```python
from build123d import *

# Parameters (mm, degrees)
SKETCH1_W           = 50
SKETCH1_H           = 40
BOSS_EXTRUDE1_DEPTH = 10
SKETCH5_W           = 6
SKETCH5_H           = 5
BOSS_EXTRUDE3_DEPTH = 10
SKETCH6_R           = 2
CUT_EXTRUDE1_DEPTH  = 20
SKETCH8_W           = 10
SKETCH8_H           = 40
CUT_EXTRUDE2_DEPTH  = 25
SKETCH12_W          = 5
SKETCH12_H          = 5
BOSS_EXTRUDE5_DEPTH = 10
SKETCH13_R          = 1.5
CUT_EXTRUDE4_DEPTH  = 10
SKETCH14_R          = 1
CUT_EXTRUDE5_DEPTH  = 10
CUT_EXTRUDE6_DEPTH  = 22
CUT_EXTRUDE7_DEPTH  = 30
CUT_EXTRUDE8_DEPTH  = 30


with BuildPart() as part:
    # Sketch1 → Boss-Extrude1 (new body)
    with BuildSketch(Plane(origin=(669.84184187, 0, 0), x_dir=(1, 0, 0), z_dir=(0, 0, 1))):
        with Locations((-671.310344828, 437.637931034)):
            Rectangle(SKETCH1_W, SKETCH1_H)
    boss_extrude1 = extrude(amount=BOSS_EXTRUDE1_DEPTH)

    # Sketch5 → Boss-Extrude3 (add)
    with BuildSketch(Plane(origin=(23.531497042, 0, 0), x_dir=(0, 0, -1), z_dir=(1, 0, 0))):
        with Locations((-5, 442.637931034)):
            Rectangle(SKETCH5_W, SKETCH5_H)
        with Locations((-5, 432.637931034)):
            Rectangle(SKETCH5_W, SKETCH5_H)
    boss_extrude3 = extrude(amount=BOSS_EXTRUDE3_DEPTH)

    # Sketch6 → Cut-Extrude1 (cut)
    with BuildSketch(Plane(origin=(669.84184187, 445.137931034, 0), x_dir=(1, 0, 0), z_dir=(0, 1, 0))):
        with Locations(Location((-641.310344828, -5, 0), (0, 0, 180))):
            Circle(SKETCH6_R)
    cut_extrude1 = extrude(amount=-CUT_EXTRUDE1_DEPTH, mode=Mode.SUBTRACT)

    # Sketch8 → Cut-Extrude2 (cut)
    with BuildSketch(Plane.ZY.offset(26.468502958)):
        with Locations((5, 437.637931034)):
            Rectangle(SKETCH8_W, SKETCH8_H)
    extrude(amount=-CUT_EXTRUDE2_DEPTH, mode=Mode.SUBTRACT)

    # Mirror1: Boss-Extrude1, Boss-Extrude3, Cut-Extrude1 across plane
    add(boss_extrude1.mirror(Plane(origin=(-1.468502958, 0, 0), x_dir=(0, 0, 1), z_dir=(1, 0, 0))))
    add(boss_extrude3.mirror(Plane(origin=(-1.468502958, 0, 0), x_dir=(0, 0, 1), z_dir=(1, 0, 0))))
    add(cut_extrude1.mirror(Plane(origin=(-1.468502958, 0, 0), x_dir=(0, 0, 1), z_dir=(1, 0, 0))), mode=Mode.SUBTRACT)

    # Sketch12 → Boss-Extrude5 (add)
    with BuildSketch(Plane(origin=(0, 457.637931034, 0), x_dir=(1, 0, 0), z_dir=(0, 1, 0))):
        with Locations((-1.468502958, -5)):
            Rectangle(SKETCH12_W, SKETCH12_H)
    extrude(amount=BOSS_EXTRUDE5_DEPTH)

    # Sketch13 → Cut-Extrude4 (cut)
    with BuildSketch(Plane(origin=(1.031497042, 0, 0), x_dir=(0, 0, -1), z_dir=(1, 0, 0))):
        with Locations((-5, 462.637931034)):
            Circle(SKETCH13_R)
    extrude(amount=-CUT_EXTRUDE4_DEPTH, mode=Mode.SUBTRACT)

    # Sketch14 → Cut-Extrude5 (cut)
    with BuildSketch(Plane.XY.offset(10)):
        with Locations((-21.468502958, 452.637931034)):
            Circle(SKETCH14_R)
        with Locations((-21.468502958, 422.637931034)):
            Circle(SKETCH14_R)
        with Locations((18.531497042, 452.637931034)):
            Circle(SKETCH14_R)
        with Locations((18.531497042, 422.637931034)):
            Circle(SKETCH14_R)
    extrude(amount=-CUT_EXTRUDE5_DEPTH, mode=Mode.SUBTRACT)

    # Sketch15 → Cut-Extrude6 (cut)
    with BuildSketch(Plane(origin=(0, 445.137931034, 0), x_dir=(1, 0, 0), z_dir=(0, 1, 0))):
        with BuildLine():
            Line((33.531497042, -2), (28.531497042, -2))
            ThreePointArc((28.531497042, -2), (30.652817386, -2.878679656), (31.531497042, -5))
            ThreePointArc((31.531497042, -5), (30.652817386, -7.121320344), (28.531497042, -8))
            Line((28.531497042, -8), (33.531497042, -8))
            Line((33.531497042, -8), (33.531497042, -2))
        make_face()
    extrude(amount=-CUT_EXTRUDE6_DEPTH, mode=Mode.SUBTRACT)

    # Sketch17 → Cut-Extrude7 (cut)
    with BuildSketch(Plane(origin=(0, 445.137931034, 0), x_dir=(1, 0, 0), z_dir=(0, 1, 0))):
        with BuildLine():
            Line((-36.468502958, -8), (-31.468502958, -8))
            ThreePointArc((-31.468502958, -8), (-34.468502958, -5), (-31.468502958, -2))
            Line((-31.468502958, -2), (-36.468502958, -2))
            Line((-36.468502958, -2), (-36.468502958, -8))
        make_face()
    extrude(amount=-CUT_EXTRUDE7_DEPTH, mode=Mode.SUBTRACT)

    # Sketch18 → Cut-Extrude8 (cut)
    with BuildSketch(Plane(origin=(1.031497042, 0, 0), x_dir=(0, 0, -1), z_dir=(1, 0, 0))):
        with BuildLine():
            Line((-7.5, 467.637931034), (-7.5, 462.637931034))
            ThreePointArc((-7.5, 462.637931034), (-5, 465.137931034), (-2.5, 462.637931034))
            Line((-2.5, 462.637931034), (-2.5, 467.637931034))
            Line((-2.5, 467.637931034), (-7.5, 467.637931034))
        make_face()
    extrude(amount=-CUT_EXTRUDE8_DEPTH, mode=Mode.SUBTRACT)


solid = part.part
```
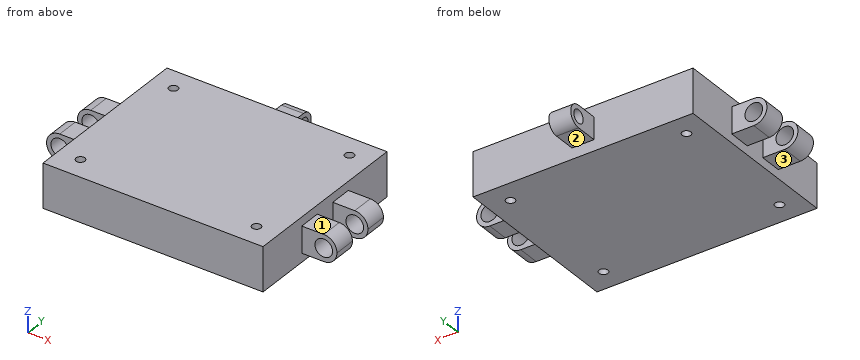
Work out the finished part from the listing and answer in its coordinate system (mm). Face numbers are marked on the shaded views. A direction names the side the tool comes from. Coordinates: 2 decimals unless noted, no trailing zeros. Loops run counter-clockwise (first coordinate to the right, second up) from the corner with the lowest first, then second, coordinate; pieces in that order, holes last. Notation, with made-up numbers: (0, -16.5) - (48, -16.5) arc R11 ccw to (48, 0.5) - close; hole circle Ø1 at (78.25, -32). An arc over 180 degrees is marked (long way). Use a Markdown table: item, result.
Item 1: Given pin 1 Ø1 at (y, z) = (460, 3.5) entering from +X; pin 2 Ø3.5 at (x, z) = (-31.47, 5) entering from +Y; pin 3 Ø5 at (x, z) = (18.5, 2) entering from +Y; pin 4 Ø5.5 at (x, y) = (27, 443) entering from +Z, each flat-ended and moving along its own axis, determine where each tip first touches the part or whether it passes through.
Evaluation:
| item | result |
|---|---|
| pin 1 | stops at x = 1.03 |
| pin 2 | passes through |
| pin 3 | stops at y = 457.64 |
| pin 4 | stops at z = 8 |
Item 2: Find section B-B, the plane y = 426. Determine the outline of the cut face in (x, z).
Evaluation:
| item | result |
|---|---|
| outline | (-26.47, 0) - (23.53, 0) - (23.53, 10) - (-26.47, 10) - close |
Item 3: For the marked faces 1, 2 and 3, determine the directions among +Z, -Z, +X, -X, +Y, -Y from which every point of the face is accessible in a straight line to the end or side of a thin tool.
Evaluation:
| item | result |
|---|---|
| face 1 | +Z, +X, +Y, -Y |
| face 2 | -Z, +X, -X, +Y |
| face 3 | -Z, -X, +Y, -Y |
Item 4: Consider probe 1 along X at (y, z) = (452, 2.5); probe 2 along Y at (x, z) = (-0.1, 5); probe 3 along X at (y, z) = (454, 1.75). Determine where each line is inside the solid, lowest interval first. Write a range as from..to.
Evaluation:
| item | result |
|---|---|
| probe 1 | x = -26.47..-22.24, -20.7..17.76, 19.3..23.53 |
| probe 2 | y = 417.64..461.14, 464.14..465.14 |
| probe 3 | x = -26.47..23.53 |
Item 5: Find section C-C, the plane x = 15. Determine the outline of the cut face in (y, z), and give its area (3 significant figures).
Evaluation:
| item | result |
|---|---|
| outline | (417.64, 0) - (457.64, 0) - (457.64, 10) - (417.64, 10) - close |
| area | 400 mm2 |
Item 6: Find section A-A, the plane y = 433.5. Determine the outline of the cut face in (x, z).
Evaluation:
| item | result |
|---|---|
| outline | (-31.47, 2) - (-26.47, 2) - (-26.47, 0) - (23.53, 0) - (23.53, 2) - (28.53, 2) arc R3 ccw to (28.53, 8) - (23.53, 8) - (23.53, 10) - (-26.47, 10) - (-26.47, 8) - (-31.47, 8) arc R3 ccw to start; hole circle Ø4 at (-31.47, 5); hole circle Ø4 at (28.53, 5) |
